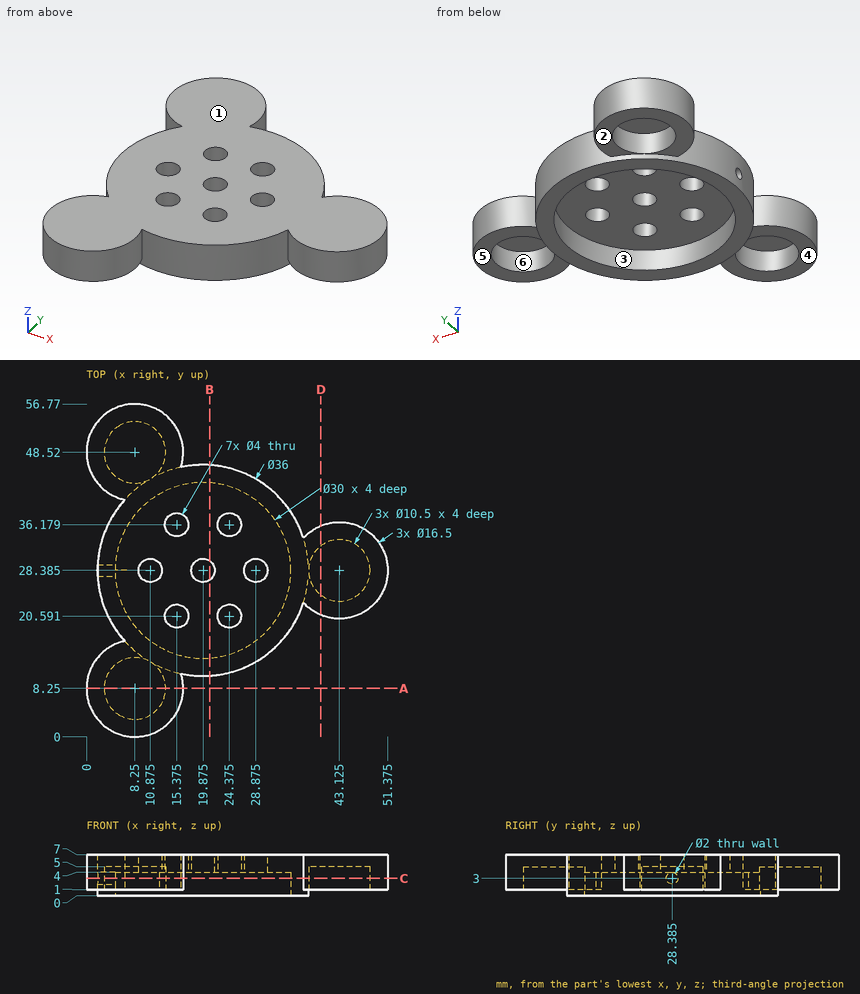
Print and shaded views of the part. All mm, measured from the part's lowest x, y and z. A direction names the side the tool comes from. Give positions to 0.01 mm unless a question says otherwise; leave off trailing zeros. Order: outer loops, then holes, each group sorted by start corner. A loop starts at its lowest first (then second) coordinate and runs counter-clockwise, first axis right, second up. Notation, with made-up numbers: (-3, -7.75) - (44, -7.75) arc R26 ccw to (44, 21.25) - close; hole circle Ø4 at (5, -38.5). An arc over 180 degrees is marked (long way). One line per item, written item: value.
Item 1: Slice it at D-D (x = 40). List the corners of the cut face in (y, z).
Response values:
outline: (20.75, 1) - (24.17, 1) - (24.17, 5) - (32.6, 5) - (32.6, 1) - (36.02, 1) - (36.02, 7) - (20.75, 7) - close
Item 2: Slice it at C-C (z = 3). Give the number of separate pieces and of enclosed holes in the cut face, then the cut area to 3 significant figures.
Response values:
separate pieces: 1
enclosed holes: 3
area: 619 mm2
Item 3: Wall check: line 1 (X direction, y = 8.25, z = 3.8); line 2 (X direction, y = 27, z = 4.75); line 3 (Y direction, x = 14, z = 5.75) (1 decimal). Give the ranges that are in metal, low to high.
Response values:
line 1: 0 to 3, 13.5 to 16.5
line 2: 1.93 to 9.43, 12.32 to 18.43, 21.32 to 27.43, 30.32 to 38.06, 48.19 to 51.26
line 3: 2.3 to 19.1, 22 to 34.7, 37.6 to 54.4
Item 4: Tool access for the marked faces 1, 2, 3 and 4: list every direction of +Z, -Z, +X, -X, +Y, -Y with a clear straight run to the whole face (end or side of a thin tool).
Response values:
face 1: +Z, +X, -X, +Y, -Y
face 2: -Z, -X, +Y
face 3: -Z
face 4: -Z, -X, -Y
Item 5: Slice it at A-A (y = 8.25). List the corners of the cut face in (x, z).
Response values:
outline: (0, 1) - (3, 1) - (3, 5) - (13.5, 5) - (13.5, 1) - (16.5, 1) - (16.5, 7) - (0, 7) - close
Item 6: Two-plate mould, pull along X, no slides. Class the marked faces 5 and 6: released by +X, released by -X, zero draft, split by the parting line, or undercut.
Response values:
face 5: zero draft
face 6: undercut
Item 7: Pin check, flat tips, straight feed: pin 1 Ø8.5 at (x, y) = (10, 6.5) entering from -Z; pin 2 Ø1.5 at (x, z) = (33, 3) entering from +Y; pin 3 Ø4.5 at (x, y) = (10.88, 28.39) entering from -Z; pin 4 Ø16 at (x, y) = (41.5, 30.5) entering from -Z. Stop position of each tip, or through.
Response values:
pin 1: z = 1
pin 2: y = 41.46
pin 3: z = 4
pin 4: z = 0
Item 8: Slice it at B-B (x = 21). List the corners of the cut face in (y, z).
Response values:
outline: (10.42, 0) - (13.43, 0) - (13.43, 4) - (26.73, 4) - (26.73, 7) - (10.42, 7) - close; (30.04, 4) - (43.34, 4) - (43.34, 0) - (46.35, 0) - (46.35, 7) - (30.04, 7) - close
